Read the model definition and answer for the solid it produces. Units are mm, in the model's axes. Give positions to 0.01 mm unless a question says otherwise; leave off trailing zeros. Order: outer loops, then holes, each group sorted by start corner. A loop starts at its lowest first (then second) coordinate and runs counter-clockwise, first axis right, second up. Notation, with made-up numbers: (49.25, 2.25) - (89.25, 2.25) arc R23 cw to (89.25, 19.25) - close; hole circle Ø7 at (33.25, -28.5). An arc over 180 degrees is marked (long way). Use a Markdown table: item, result. Add a question column.
1. A cutting plane is placed at A-A on x = -86. Determine the outline of the cut face in (y, z).
2. For a pull along X with two mould halves and no side action, classify faces 1 (the cylindrical face through (136.397, 42.953, -21.199)), 2 (the cylindrical face through (-120.94, -92.73, -21.2)), 3 (the flat face through (-136.2, -44.4, 0)) as released by +X, released by -X, zero draft, split by the parting line, or undercut.
3. A cutting plane is placed at B-B on y = -83. Determine the outline of the cut face in (x, z).
4. A cutting plane is placed at C-C on z = -22. State how many separate pieces and enclosed holes the cut face has, and give its area (3 significant figures).
5. Consider L1, parallel to X at y = -58, z = -28.5; L2, parallel to Y at x = 60.5, z = -13.5; L3, parallel to X at y = -108, z = -6. Determine where each line is inside the solid, lowest interval first.
6. Flat-ended cylindrical pins translate along their axes: P1, Ø8, axis at x = 93.5, z = -31, coming from the +Y side; P2, Ø10, axis at x = 108.5, z = -12.5, coming from the -Y side; P3, Ø1.5, axis at y = -89.5, z = -27.5, coming from the +X side. Find the tip coordinate at first contact, or state that the pin passes through.
```python
from build123d import *

# Parameters (mm, degrees)
SKETCH1_R           = 152.4
SKETCH1_R_2         = 143
BOSS_EXTRUDE1_DEPTH = 43
CUT_EXTRUDE1_DEPTH  = 220.773792796
CIRPATTERN1_COUNT   = 16


with BuildPart() as part:
    # Sketch1 → Boss-Extrude1 (new body)
    with BuildSketch(Plane(origin=(0, 0, 0), x_dir=(0, 1, 0), z_dir=(0, 0, 1))):
        with Locations(Location((0, 0, 0), (0, 0, 270))):
            Circle(SKETCH1_R)
        with Locations(Location((0, 0, 0), (0, 0, 270))):
            Circle(SKETCH1_R_2, mode=Mode.SUBTRACT)
    extrude(amount=-BOSS_EXTRUDE1_DEPTH)

    # Sketch1_3 → Cut-Extrude1 (cut, through all)
    with BuildSketch(Plane(origin=(0, 0, 0), x_dir=(0, 1, 0), z_dir=(0, 0, 1))):
        with BuildLine():
            ThreePointArc((0, 150.1892), (-2.4892, 147.7), (0, 145.2108))
            Line((0, 145.2108), (0, 150.1892))
        make_face()
        with BuildLine():
            Line((0, 150.1892), (0, 145.2108))
            ThreePointArc((0, 145.2108), (1.7601302, 145.9398698), (2.4892, 147.7))
            ThreePointArc((2.4892, 147.7), (1.7601302, 149.4601302), (0, 150.1892))
        make_face()
    cut_extrude1 = extrude(amount=-CUT_EXTRUDE1_DEPTH, mode=Mode.SUBTRACT)

    # CirPattern1: Cut-Extrude1 ×16 about axis
    cirpattern1_axis = Axis((0, 0, 0), (0, 0, 1))
    for i in range(1, CIRPATTERN1_COUNT):
        add(cut_extrude1.rotate(cirpattern1_axis, i * 360 / CIRPATTERN1_COUNT), mode=Mode.SUBTRACT)


solid = part.part
```
Output values:
| question | item | result |
|---|---|---|
| 1 | outline | (-125.82, -43) - (-114.25, -43) - (-114.25, 0) - (-125.82, 0) - close; (114.25, -43) - (125.82, -43) - (125.82, 0) - (114.25, 0) - close |
| 2 | face 1 | undercut |
| 2 | face 2 | split by the parting line |
| 2 | face 3 | zero draft |
| 3 | outline | (-127.82, -43) - (-116.45, -43) - (-116.45, 0) - (-127.82, 0) - close; (116.45, -43) - (127.82, -43) - (127.82, 0) - (116.45, 0) - close |
| 4 | separate pieces | 1 |
| 4 | enclosed holes | 17 |
| 4 | area | 8,410 mm² |
| 5 | L1 | -140.93 to -138.46, -134.45 to -130.71, 130.71 to 134.45, 138.46 to 140.93 |
| 5 | L2 | -139.88 to -129.57, 129.57 to 139.88 |
| 5 | L3 | -107.53 to -93.73, 93.73 to 107.53 |
| 6 | P1 | y = 123.35 |
| 6 | P2 | y = -111.86 |
| 6 | P3 | x = 123.89 |
